Check sheet for the modelled part. Datum: model origin and axes. Units: mm. A direction names the side the tool comes from. Round coordinates to 2 decimals unless told otherwise and drop trailing zeros. Order: outer loops, then holes, each group sorted by start corner. A loop starts at its lowest first (then second) coordinate and runs counter-clockwise, first axis right, second up. Notation, with made-up numbers: (13, -5) -> (53, -5) arc R24 cw to (53, 24) -> close; hole circle Ø7 at (61.25, 8.25). An arc over 180 degrees is marked (long way). Answer in a Markdown table with one row per item.
```python
from build123d import *

# Parameters (mm, degrees)
SKETCH_1_W          = 25
SKETCH_1_H          = 31
EXTRUDE_1_DEPTH     = 2
SKETCH_2_W          = 21.5
SKETCH_2_H          = 27.5
EXTRUDE_2_DEPTH     = 27
SKETCH_3_W          = 19
SKETCH_3_H          = 24
EXTRUDE_3_DEPTH     = 4
CUT_EXTRUDE_START   = -19
CUT_EXTRUDE_1_DEPTH = 19
SKETCH_6_W          = 21.5
SKETCH_6_H          = 27.5
SKETCH_6_W_2        = 1.2
SKETCH_6_H_2        = 25
SKETCH_6_W_3        = 6.5
SKETCH_6_H_3        = 0.8
CUT_EXTRUDE_2_DEPTH = 11


# Read off the part's stored shape, not the designer's step: 切除-拉伸1
with BuildPart() as part:
    # 草图1 → 拉伸1 (new body)
    with BuildSketch(Plane.XY):
        Rectangle(SKETCH_1_W, SKETCH_1_H)
    extrude(amount=EXTRUDE_1_DEPTH)

    # 草图2 → 拉伸2 (add)
    with BuildSketch(Plane.XY.offset(2)):
        Rectangle(SKETCH_2_W, SKETCH_2_H)
    extrude(amount=EXTRUDE_2_DEPTH)

    # 草图3 → 拉伸3 (add)
    with BuildSketch(Plane(origin=(0, 0, 0), x_dir=(-1, 0, 0), z_dir=(0, 0, -1))):
        Rectangle(SKETCH_3_W, SKETCH_3_H)
    extrude(amount=EXTRUDE_3_DEPTH)

    # 切除-拉伸1 outline → 切除-拉伸1 (cut)
    with BuildSketch(Plane.ZY.offset(9.5).offset(CUT_EXTRUDE_START)):
        with BuildLine():
            Line((-4, -12), (-0.39560665, -12))
            add(Edge.make_bspline(
                [(-0.39560665, -12), (-0.407203251, -10.938807734), (-0.456034027, -6.470357075), (-1.244501589, 1.361302539), (-3.086230941, 7.87953286), (-4, 11.113535286)],
                knots=[0, 0, 0, 0, 0.135639857, 0.571150042, 1, 1, 1, 1], degree=3))
            Line((-4, 11.113535286), (-4, -12))
        make_face()
        with BuildLine():
            Line((-4, 12), (-4, 11.113535286))
            add(Edge.make_bspline(
                [(-4, 11.113535286), (-3.189353387, 11.383960845), (-1.884330596, 11.819306546), (-0.517710732, 11.950355346), (0, 12)],
                knots=[0, 0, 0, 0, 0.621174296, 1, 1, 1, 1], degree=3))
            Line((0, 12), (-4, 12))
        make_face()
    extrude(amount=CUT_EXTRUDE_1_DEPTH, mode=Mode.SUBTRACT)

    # 草图6 → 切除-拉伸2 (cut)
    with BuildSketch(Plane.XY.offset(29)):
        Rectangle(SKETCH_6_W, SKETCH_6_H)
        Rectangle(SKETCH_6_W_2, SKETCH_6_H_2, mode=Mode.SUBTRACT)
        with Locations((-5.5, 9.5)):
            Rectangle(SKETCH_6_W_3, SKETCH_6_H_3, mode=Mode.SUBTRACT)
        with Locations((5.5, 9.5)):
            Rectangle(SKETCH_6_W_3, SKETCH_6_H_3, mode=Mode.SUBTRACT)
        with Locations((-5.5, 0)):
            Rectangle(SKETCH_6_W_3, SKETCH_6_H_3, mode=Mode.SUBTRACT)
        with Locations((5.5, 0)):
            Rectangle(SKETCH_6_W_3, SKETCH_6_H_3, mode=Mode.SUBTRACT)
    extrude(amount=-CUT_EXTRUDE_2_DEPTH, mode=Mode.SUBTRACT)


solid = part.part
```
(1) Depth check by flat-ended pin: pin 1 Ø8 at (y, z) = (9.5, 17) entering from -X; pin 2 Ø5 at (y, z) = (-6, 9) entering from +X; pin 3 Ø0.6 at (y, z) = (9.5, 22.5) entering from +X; pin 4 Ø4.5 at (y, z) = (5.5, -1.5) entering from +X. Enter the tip coordinate at first touch or a pass-through.
Solutions:
| item | result |
|---|---|
| pin 1 | x = -10.75 |
| pin 2 | x = 10.75 |
| pin 3 | x = 8.75 |
| pin 4 | x = 12.5 |
(2) Section check B-B on z = 16. Record the boundary of the cut face in (x, y), plus the area to 3 significant figures.
Solutions:
| item | result |
|---|---|
| outline | (-10.75, -13.75) -> (10.75, -13.75) -> (10.75, 13.75) -> (-10.75, 13.75) -> close |
| area | 591 mm^2 |
(3) Scan lines: probe 1 along Y at (x, z) = (-7.25, 20); probe 2 along X at (y, z) = (2.5, 20); probe 3 along X at (y, z) = (-3, 14.5). Record each from-to range of solid material in increasing order. Write a range as from..to.
Solutions:
| item | result |
|---|---|
| probe 1 | -0.4..0.4, 9.1..9.9 |
| probe 2 | -0.6..0.6 |
| probe 3 | -10.75..10.75 |
(4) Section check A-A on z = 25.5. Record the boundary of the cut face in (x, y).
Solutions:
| item | result |
|---|---|
| outline | (-8.75, -0.4) -> (-2.25, -0.4) -> (-2.25, 0.4) -> (-8.75, 0.4) -> close; (-8.75, 9.1) -> (-2.25, 9.1) -> (-2.25, 9.9) -> (-8.75, 9.9) -> close; (-0.6, -12.5) -> (0.6, -12.5) -> (0.6, 12.5) -> (-0.6, 12.5) -> close; (2.25, -0.4) -> (8.75, -0.4) -> (8.75, 0.4) -> (2.25, 0.4) -> close; (2.25, 9.1) -> (8.75, 9.1) -> (8.75, 9.9) -> (2.25, 9.9) -> close |
(5) Tool access check on faces 1 (the flat face through (0, 13.75, 10)), 2 (the flat face through (5, -0.4, 24)), 3 (the flat face through (0, -12.5, 24)), 4 (the flat face through (5, 9.1, 24)), 5 (the flat face through (-9.5, 5, -1)). Record the directions out of +Z, -Z, +X, -X, +Y, -Y that give a thin tool (end or side, any length) a straight path to the whole face; none if there is none.
Solutions:
| item | result |
|---|---|
| face 1 | +Z, +X, -X, +Y |
| face 2 | +Z, +X, -Y |
| face 3 | +Z, +X, -X, -Y |
| face 4 | +Z, +X |
| face 5 | -Z, -X, +Y, -Y |
(6) Draft check along X on faces 6 (the flat face through (-10.75, 0, 10)), 7 (the flat face through (-2.25, 9.5, 23.6)), 8 (the flat face through (8.75, 9.5, 23.6)), 9 (the flat face through (5, 9.9, 24)). Enter one of: pulls with the +X half, pulls with the -X half, needs draft (parallel to the pull), parting line crosses it, or undercut.
Solutions:
| item | result |
|---|---|
| face 6 | pulls with the -X half |
| face 7 | undercut |
| face 8 | pulls with the +X half |
| face 9 | needs draft |
